Here's how the part is built. I have some questions about the finished solid (model axes, mm). Give positions to 0.01 mm unless a question says otherwise; leave off trailing zeros. Loops run counter-clockwise (first coordinate to the right, second up) from the corner with the lowest first, then second, coordinate; pieces in that order, holes last.
Q1. If we section it at B-B (z = -19.5): Please give me the cut outline in (x, y).
Q2. I need wall thicknesses on line 1 (Z direction, x = -30, y = 1.3); line 2 (Z direction, x = -29.21, y = 0.8) (3 decimals); line 3 (X direction, y = 1.55, z = 16). Which ranges of each line are inside material? Lowest first, please.
Q3. If we section it at A-A (y = 0.5): Give the number of separate pieces and of enclosed holes in the cut face, plus the area to 3 significant figures.
Q4. Will this pin go through, and if not, where does the flat tip stop? P1, Ø2, axis at x = 30, z = 17.202, coming from the +Y side.
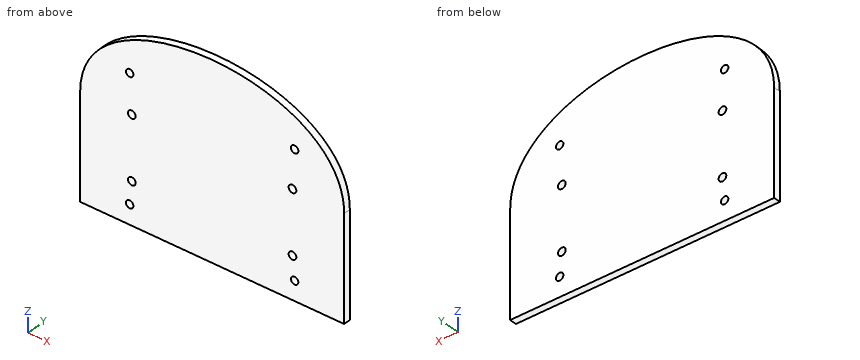
from build123d import *

# Parameters (mm, degrees)
BOSS_EXTRUDE1_DEPTH     = 2.54
CUT_EXTRUDE1_DEPTH      = 60.34583774
CUT_EXTRUDE1_DEPTH_BACK = 60.34583774
SKETCH3_R               = 1.35
SKETCH3_R_2             = 1.397


with BuildPart() as part:
    # Sketch2 → Boss-Extrude1 (new body)
    with BuildSketch(Plane(origin=(0, 0, 0), x_dir=(1, 0, 0), z_dir=(0, 1, 0))):
        with BuildLine():
            Line((48.006, 34.798), (-48.006, 34.798))
            Line((-48.006, 34.798), (-48.006, -3.048))
            add(Edge.make_bspline(
                [(-48.006, -3.048), (-48.006, -45.381333333), (48.006, -45.381333333), (48.006, -3.048)],
                knots=[0, 0, 0, 0, 1, 1, 1, 1], degree=3))
            Line((48.006, -3.048), (48.006, 34.798))
        make_face()
    extrude(amount=BOSS_EXTRUDE1_DEPTH)

    # Sketch3 → Cut-Extrude1 (cut, two sides: drawn at the far end of the back side and taken through both)
    with BuildSketch(Plane(origin=(0, 2.54, 0), x_dir=(1, 0, 0), z_dir=(0, 1, 0)).offset(-CUT_EXTRUDE1_DEPTH_BACK)):
        with Locations(Location((-30, 27.798, 0), (0, 0, 270))):
            Circle(SKETCH3_R)
        with Locations(Location((-30, -17.202, 0), (0, 0, 270))):
            Circle(SKETCH3_R)
        with Locations(Location((30, -17.202, 0), (0, 0, 90))):
            Circle(SKETCH3_R)
        with Locations(Location((30, 27.798, 0), (0, 0, 90))):
            Circle(SKETCH3_R)
        with Locations(Location((-29.21, 19.558, 0), (0, 0, 270))):
            Circle(SKETCH3_R_2)
        with Locations(Location((-29.21, -3.302, 0), (0, 0, 270))):
            Circle(SKETCH3_R_2)
        with Locations(Location((29.21, -3.302, 0), (0, 0, 90))):
            Circle(SKETCH3_R_2)
        with Locations(Location((29.21, 19.558, 0), (0, 0, 90))):
            Circle(SKETCH3_R_2)
    extrude(amount=CUT_EXTRUDE1_DEPTH + CUT_EXTRUDE1_DEPTH_BACK, mode=Mode.SUBTRACT)


solid = part.part
Check sheet entries:
1. outline: (-48.01, 0) - (-30.61, 0) - (-30.61, 2.54) - (-48.01, 2.54) - close; (-27.81, 0) - (27.81, 0) - (27.81, 2.54) - (-27.81, 2.54) - close; (30.61, 0) - (48.01, 0) - (48.01, 2.54) - (30.61, 2.54) - close
2. line 1: z = -34.8 to -29.15, -26.45 to -20.71, -18.41 to 2.15, 4.45 to 15.85, 18.55 to 28.48
2. line 2: z = -34.798 to -28.893, -26.703 to -20.955, -18.161 to 1.905, 4.699 to 16.107, 18.297 to 28.855
2. line 3: x = -44.47 to -30.61, -29.39 to 29.39, 30.61 to 44.47
3. separate pieces: 1
3. enclosed holes: 8
3. area: 6,020 mm2
4. P1: passes through
